from build123d import *

# Parameters (mm, degrees)
SKETCH1_W           = 50
SKETCH1_H           = 55
BOSS_EXTRUDE1_DEPTH = 50
SKETCH2_W           = 50
SKETCH2_H           = 50
CUT_EXTRUDE1_DEPTH  = 45
FILLET2_R           = 10


with BuildPart() as part:
    # Sketch1 → Boss-Extrude1 (new body)
    with BuildSketch(Plane.XY):
        with Locations((9.585987261, 0.398089172)):
            Rectangle(SKETCH1_W, SKETCH1_H)
    extrude(amount=BOSS_EXTRUDE1_DEPTH)

    # Sketch2 → Cut-Extrude1 (cut)
    with BuildSketch(Plane.XY.offset(50)):
        with Locations((9.585987261, 2.898089172)):
            Rectangle(SKETCH2_W, SKETCH2_H)
    extrude(amount=-CUT_EXTRUDE1_DEPTH, mode=Mode.SUBTRACT)

    # Fillet2
    fillet2_edges = [part.edges().sort_by_distance(p)[0] for p in [
        (9.585987261, -27.101910828, 0),
    ]]
    fillet(fillet2_edges, radius=FILLET2_R)


solid = part.part
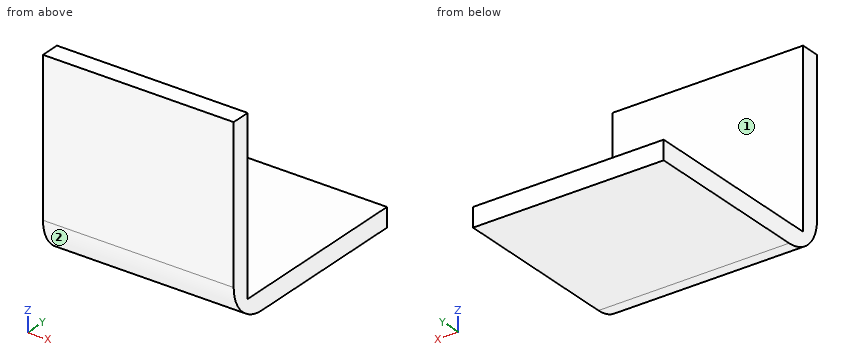
The listing builds one solid part. Answer for the finished solid, in the listing's coordinates (mm). Face numbers are marked on the shaded views. A direction names the side the tool comes from. Coordinates: 2 decimals unless noted, no trailing zeros. Loops run counter-clockwise (first coordinate to the right, second up) from the corner with the lowest first, then second, coordinate; pieces in that order, holes last.
1) Find section A-A on x = 12.5. Write down the section's boundary in (y, z), then the cut area to 3 significant figures.
2) Flat-ended cylindrical pins translate along their axes: pin 1 Ø8 at (x, z) = (28.5, 19.5) entering from +Y; pin 2 Ø10 at (x, y) = (10.5, 10) entering from +Z. Find the tip coordinate at first contact, or state that the pin passes through.
3) Find section C-C on y = 23. Write down the section's boundary in (x, z).
4) A tool of negligible diameter and unlimited length cuts with its end or side. For the marked faces 1 and 2, from which of +Z, -Z, +X, -X, +Y, -Y can it reach the whole face along a straight path? Write none if from no direction.
5) Find the intervals of material crossed by L1, parallel to Y at x = 26.5, z = 15; L2, parallel to Z at x = 9, y = -14; L3, parallel to Z at x = 13.5, y = -24, in increasing order.
6) Find section B-B on z = 11.5. Write down the section's boundary in (x, y).
Values:
1. outline: (-27.1, 10) arc R10 ccw to (-17.1, 0) - (27.9, 0) - (27.9, 5) - (-22.1, 5) - (-22.1, 50) - (-27.1, 50) - close
1. area: 479 mm2
2. pin 1: stops at y = -22.1
2. pin 2: stops at z = 5
3. outline: (-15.41, 0) - (34.59, 0) - (34.59, 5) - (-15.41, 5) - close
4. face 1: +Z, +X, -X, +Y
4. face 2: -Z, +X, -X, -Y
5. L1: y = -27.1 to -22.1
5. L2: z = 0 to 5
5. L3: z = 2.76 to 50
6. outline: (-15.41, -27.1) - (34.59, -27.1) - (34.59, -22.1) - (-15.41, -22.1) - close
